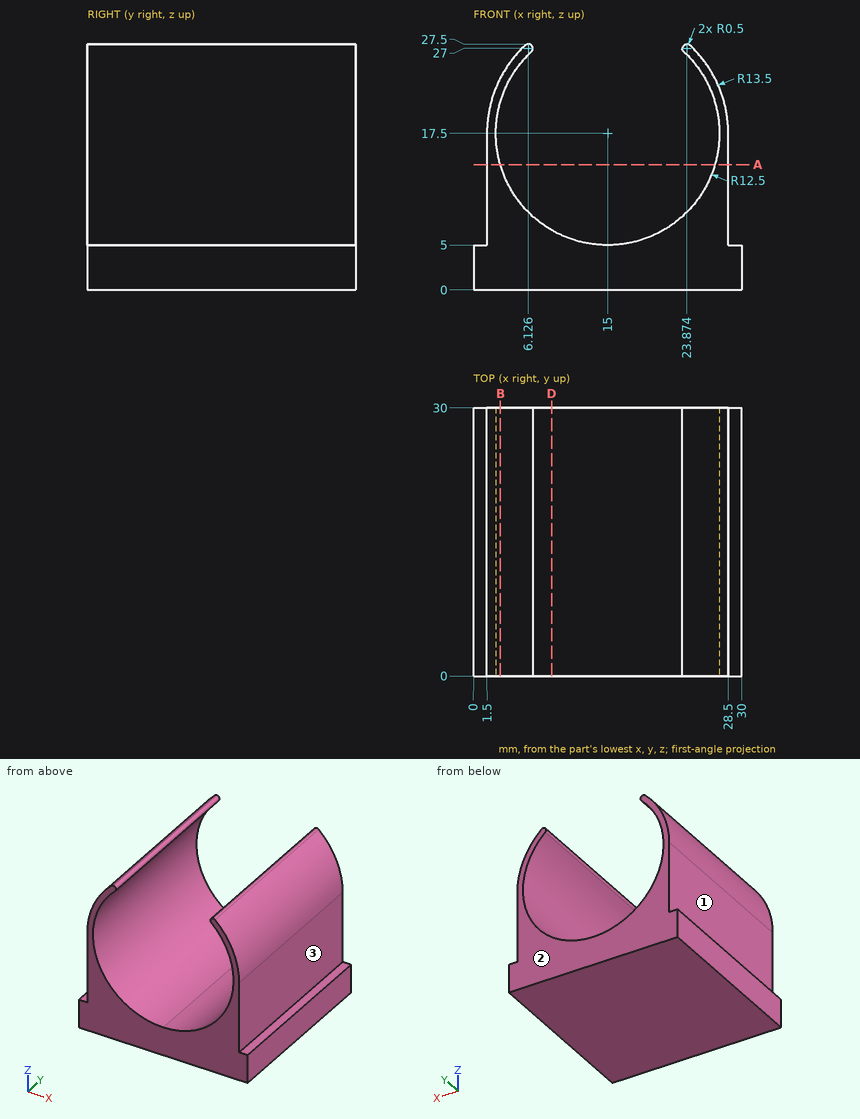
Input: dimensioned drawing with shaded views. Units: mm. Origin: part minimum x, y, z. A direction names the side the tool comes from. Round coordinates to 2 decimals unless told otherwise and drop trailing zeros. Loops run counter-clockwise (first coordinate to the right, second up) from the corner with the lowest first, then second, coordinate; pieces in that order, holes last. Notation, with made-up numbers: (48.5, -4) -> (73.5, -4) arc R31 cw to (73.5, 23) -> close; hole circle Ø2 at (40.5, 63). An arc over 180 degrees is marked (long way). Answer as a JSON object with one key per item and string values. Group by question number.
Q1. Section query A-A (z = 14). Output: boundary loops of the cut face in (x, y).
Q2. Access query for the marked faces 1, 2 and 3. Directions: +Z, -Z, +X, -X, +Y, -Y. A direction counts if a zero-diameter tool reaches every point of the face in a straight line with its end or side. Return the directions, or none.
Q3. Ray query, line 1 (X direction, y = 21, z = 25) (1 decimal); line 2 (X direction, y = 3, z = 15.5); line 3 (Z direction, x = 25.5, y = 24.5) (1 decimal). Return the intervals inside material, ascending. Write a range as from..to.
Q4. Section query D-D (x = 8.75). Output: boundary loops of the cut face in (y, z), plus the area to 3 significant figures.
Q5. Section query B-B (x = 3). Output: boundary loops of the cut face in (y, z).
Q6. Contact query for flat-ended pins moving along their axis: P1, Ø2, axis at x = 4.5, y = 18, coming from the +Z side; P2, Ø12, axis at y = 25.5, z = 22.5, coming from the +X side; P3, Ø6, axis at y = 16, z = 10.5, coming from the -X side; P4, Ø6, axis at x = 22.5, z = 12.5, coming from the +Y side. Output: stop coordinate, or through.
Completed:
{
 "1": {"outline": "(1.5, 0) -> (3, 0) -> (3, 30) -> (1.5, 30) -> close; (27, 0) -> (28.5, 0) -> (28.5, 30) -> (27, 30) -> close"},
 "2": {"face 1": "+Z, -X, +Y, -Y", "face 2": "+Z, -Z, +X, -X, +Y", "face 3": "+Z, +X, +Y, -Y"},
 "3": {"line 1": "3.8..5, 25..26.2", "line 2": "1.5..2.66, 27.34..28.5", "line 3": "0..10.7, 24.3..26"},
 "4": {"outline": "(0, 0) -> (30, 0) -> (30, 6.67) -> (0, 6.67) -> close", "area": "200 mm²"},
 "5": {"outline": "(0, 0) -> (30, 0) -> (30, 14) -> (0, 14) -> close; (0, 21) -> (30, 21) -> (30, 23.68) -> (0, 23.68) -> close"},
 "6": {"P1": "z = 27.09", "P2": "x = 28.5", "P3": "x = 1.5", "P4": "through"}
}
